from build123d import *

# Parameters (mm, degrees)
F0_R     = 1.6
F0_R_2   = 2
F1_DEPTH = 3.175


# Not quite as in the source:
# - a length typed as a fraction of an inch, garbled in the dataset ("3 / 203.2 mm" for 3/8 in), is restored


with BuildPart() as f1:
    # F0 (on Front) → F1 (new body)
    with BuildSketch(Plane.XZ):
        with BuildLine():
            Line((26.215, 8.975), (-6.165, 8.975))
            ThreePointArc((-6.165, 8.975), (-8.8590768363, 7.8590768363), (-9.975, 5.165))
            Line((-9.975, 5.165), (-9.975, -47.215))
            ThreePointArc((-9.975, -47.215), (-8.8590768363, -49.9090768363), (-6.165, -51.025))
            Line((-6.165, -51.025), (26.215, -51.025))
            ThreePointArc((26.215, -51.025), (28.9090768363, -49.9090768363), (30.025, -47.215))
            Line((30.025, -47.215), (30.025, 5.165))
            ThreePointArc((30.025, 5.165), (28.9090768363, 7.8590768363), (26.215, 8.975))
        make_face()
        with Locations((-4.975, -46.025)):
            Circle(F0_R, mode=Mode.SUBTRACT)
        with Locations((5.1, -46.025)):
            Circle(F0_R_2, mode=Mode.SUBTRACT)
        with Locations((-4.975, -36.025)):
            Circle(F0_R, mode=Mode.SUBTRACT)
        with Locations((-4.975, -26.025)):
            Circle(F0_R, mode=Mode.SUBTRACT)
        Polygon((0, -41), (0, 0), (20.025, 0), (20.025, -41.025), (12.4728614733, -41.025), (12.4728614733, -48.485), (7.5228614733, -48.485), (7.5228614733, -41.025), align=None, mode=Mode.SUBTRACT)
        with Locations((14.9, -46.025)):
            Circle(F0_R_2, mode=Mode.SUBTRACT)
        with Locations((25, -46.025)):
            Circle(F0_R, mode=Mode.SUBTRACT)
        with Locations((25, -36.025)):
            Circle(F0_R, mode=Mode.SUBTRACT)
        with Locations((25, -26.025)):
            Circle(F0_R, mode=Mode.SUBTRACT)
        with Locations((-4.975, -16.025)):
            Circle(F0_R, mode=Mode.SUBTRACT)
        with Locations((-4.975, -6.025)):
            Circle(F0_R, mode=Mode.SUBTRACT)
        with Locations((-4.975, 3.975)):
            Circle(F0_R, mode=Mode.SUBTRACT)
        with Locations((5.125, 3.975)):
            Circle(F0_R_2, mode=Mode.SUBTRACT)
        with Locations((25, -16.025)):
            Circle(F0_R, mode=Mode.SUBTRACT)
        with Locations((14.925, 3.975)):
            Circle(F0_R_2, mode=Mode.SUBTRACT)
        with Locations((25, -6.025)):
            Circle(F0_R, mode=Mode.SUBTRACT)
        with Locations((25, 3.975)):
            Circle(F0_R, mode=Mode.SUBTRACT)
    extrude(amount=F1_DEPTH)


solid = f1.part
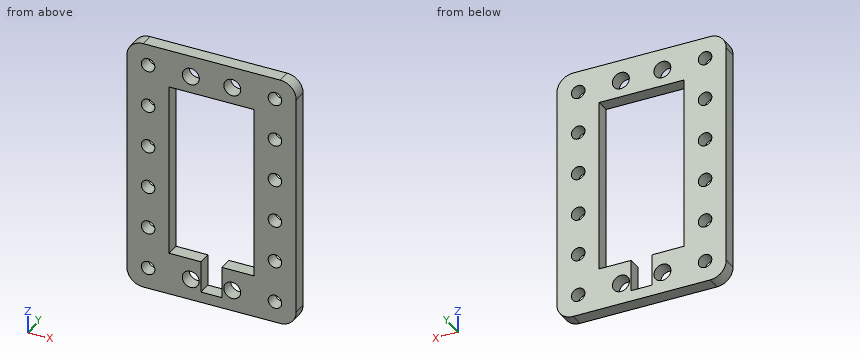
Build history of the part. All positions in model axes, mm. Round coordinates to 2 decimals unless told otherwise and drop trailing zeros. Write each loop counter-clockwise with the first axis right and the second up, starting at its lowest first coordinate (ties: lowest second). Pieces come first, ordered by that corner, then holes. Notation, with made-up numbers: (55, -37) - (79, -37) arc R22 cw to (79, -17) - close; hole circle Ø4 at (-28.5, -24.5). An arc over 180 degrees is marked (long way). One line per question, with ' | ' between items.
1. Band-saw the part on B-B, the plane z = -20. Write the cut outline in (x, y) (3 decimals), and give its area (3 significant figures).
Results are:
outline: (-9.975, -3.175) - (0, -3.175) - (0, 0) - (-9.975, 0) - close; (20.025, -3.175) - (30.025, -3.175) - (30.025, 0) - (20.025, 0) - close | area: 63.4 mm^2
2. Band-saw the part on A-A, the plane x = 25. Write the cut outline in (y, z) (3 decimals).
Results are:
outline: (-3.175, -51.025) - (0, -51.025) - (0, -47.625) - (-3.175, -47.625) - close; (-3.175, -44.425) - (0, -44.425) - (0, -37.625) - (-3.175, -37.625) - close; (-3.175, -34.425) - (0, -34.425) - (0, -27.625) - (-3.175, -27.625) - close; (-3.175, -24.425) - (0, -24.425) - (0, -17.625) - (-3.175, -17.625) - close; (-3.175, -14.425) - (0, -14.425) - (0, -7.625) - (-3.175, -7.625) - close; (-3.175, -4.425) - (0, -4.425) - (0, 2.375) - (-3.175, 2.375) - close; (-3.175, 5.575) - (0, 5.575) - (0, 8.975) - (-3.175, 8.975) - close
3. Drill centre lines: line 1 along Z through (x, y) = (14.9, -0.75) (3 decimals); line 2 along X through (y, z) = (-1.6, -43) (3 decimals); line 3 along X through (y, z) = (-2.8, -35) (3 decimals). Where is each one in solid material? Low to high. Write a range as from..to.
Results are:
line 1: -51.025..-48.025, -44.025..-41.025, 0..1.975, 5.975..8.975 | line 2: -9.975..7.523, 12.473..30.025 | line 3: -9.975..-6.204, -3.746..0, 20.025..23.771, 26.229..30.025
4. Band-saw the part on C-C, the plane x = 19. Write the cut outline in (y, z) (3 decimals).
Results are:
outline: (-3.175, -51.025) - (0, -51.025) - (0, -41.025) - (-3.175, -41.025) - close; (-3.175, 0) - (0, 0) - (0, 8.975) - (-3.175, 8.975) - close
5. Band-saw the part on D-D, the plane x = 5.1. Write the cut outline in (y, z) (3 decimals).
Results are:
outline: (-3.175, -51.025) - (0, -51.025) - (0, -48.025) - (-3.175, -48.025) - close; (-3.175, -44.025) - (0, -44.025) - (0, -41.017) - (-3.175, -41.017) - close; (-3.175, 0) - (0, 0) - (0, 1.975) - (-3.175, 1.975) - close; (-3.175, 5.975) - (0, 5.975) - (0, 8.975) - (-3.175, 8.975) - close
